from build123d import *

# Parameters (mm, degrees)
SKETCH_2_W           = 80
SKETCH_2_H           = 34
SKETCH_2_R           = 4.05
EXTRUDE_1_DEPTH      = 8
SKETCH_3_R           = 2.55
CUT_EXTRUDE_1_DEPTH  = 88.292611371
CUT_EXTRUDE_2_DEPTH  = 88.292611371
SKETCH_5_R           = 1.55
CUT_EXTRUDE_3_DEPTH  = 88.292611371
CUT_EXTRUDE_4_DEPTH  = 4.5
CUT_EXTRUDE_5_DEPTH  = 4.5
SKETCH_20_R          = 5.5
CUT_EXTRUDE_12_DEPTH = 4.5
CUT_EXTRUDE_11_DEPTH = 2
EXTRUDE_2_DEPTH      = 8


with BuildPart() as part:
    # 草图2 → 凸台-拉伸1 (new body)
    with BuildSketch(Plane.XY):
        with Locations((40, 17)):
            Rectangle(SKETCH_2_W, SKETCH_2_H)
        with Locations((7, 8)):
            Circle(SKETCH_2_R, mode=Mode.SUBTRACT)
        with Locations((40, 10)):
            Circle(SKETCH_2_R, mode=Mode.SUBTRACT)
        with Locations((73, 8)):
            Circle(SKETCH_2_R, mode=Mode.SUBTRACT)
    extrude_1 = extrude(amount=EXTRUDE_1_DEPTH)

    # 草图3 → 切除-拉伸1 (cut, through all)
    with BuildSketch(Plane.XY.offset(8)):
        with Locations((23, 8)):
            Circle(SKETCH_3_R)
        with Locations((57, 8)):
            Circle(SKETCH_3_R)
    cut_extrude_1 = extrude(amount=-CUT_EXTRUDE_1_DEPTH, mode=Mode.SUBTRACT)

    # 草图4 → 切除-拉伸2 (cut, through all)
    with BuildSketch(Plane(origin=(80, 0, 0), x_dir=(0, 0, -1), z_dir=(1, 0, 0))):
        Polygon((-1.5, 32.2), (-2.5, 32.2), (-2.5, 34), (0, 34), (0, 28.8), (-1.5, 28.8), align=None)
    cut_extrude_2 = extrude(amount=-CUT_EXTRUDE_2_DEPTH, mode=Mode.SUBTRACT)

    # 草图5 → 切除-拉伸3 (cut, through all)
    with BuildSketch(Plane.XY.offset(8)):
        with Locations((48, 10)):
            Circle(SKETCH_5_R)
        with Locations((32, 10)):
            Circle(SKETCH_5_R)
    cut_extrude_3 = extrude(amount=-CUT_EXTRUDE_3_DEPTH, mode=Mode.SUBTRACT)

    # 草图7 → 切除-拉伸4 (cut)
    with BuildSketch(Plane(origin=(0, 0, 0), x_dir=(-1, 0, 0), z_dir=(0, 0, -1))):
        with BuildLine():
            Line((-27.05, 10), (-27.05, 2.5))
            ThreePointArc((-27.05, 2.5), (-27.782233047, 0.732233047), (-29.55, 0))
            Line((-29.55, 0), (-16.45, 0))
            ThreePointArc((-16.45, 0), (-18.217766953, 0.732233047), (-18.95, 2.5))
            Line((-18.95, 2.5), (-18.95, 10))
            ThreePointArc((-18.95, 10), (-23, 14.05), (-27.05, 10))
        make_face()
        with BuildLine():
            Line((-61.05, 2.5), (-61.05, 10))
            ThreePointArc((-61.05, 10), (-57, 14.05), (-52.95, 10))
            Line((-52.95, 10), (-52.95, 2.5))
            ThreePointArc((-52.95, 2.5), (-52.217766953, 0.732233047), (-50.45, 0))
            Line((-50.45, 0), (-63.55, 0))
            ThreePointArc((-63.55, 0), (-61.782233047, 0.732233047), (-61.05, 2.5))
        make_face()
    cut_extrude_4 = extrude(amount=-CUT_EXTRUDE_4_DEPTH, mode=Mode.SUBTRACT)

    # 草图8 → 切除-拉伸5 (cut)
    with BuildSketch(Plane(origin=(0, 0, 0), x_dir=(-1, 0, 0), z_dir=(0, 0, -1))):
        with BuildLine():
            Line((-30.5, 12.85), (-49.5, 12.85))
            ThreePointArc((-49.5, 12.85), (-52.35, 10), (-49.5, 7.15))
            Line((-49.5, 7.15), (-30.5, 7.15))
            ThreePointArc((-30.5, 7.15), (-27.65, 10), (-30.5, 12.85))
        make_face()
    cut_extrude_5 = extrude(amount=-CUT_EXTRUDE_5_DEPTH, mode=Mode.SUBTRACT)

    # 草图20 → 切除-拉伸12 (cut)
    with BuildSketch(Plane(origin=(0, 0, 0), x_dir=(-1, 0, 0), z_dir=(0, 0, -1))):
        with Locations((-40, 10)):
            Circle(SKETCH_20_R)
    cut_extrude_12 = extrude(amount=-CUT_EXTRUDE_12_DEPTH, mode=Mode.SUBTRACT)

    # 草图19 → 切除-拉伸11 (cut)
    with BuildSketch(Plane(origin=(0, 0, 2.5), x_dir=(-1, 0, 0), z_dir=(0, 0, -1))):
        with BuildLine():
            Line((-25, 34), (-55.247938178, 34))
            Line((-55.247938178, 34), (-55.247938178, 33.2))
            ThreePointArc((-55.247938178, 33.2), (-54.747938178, 32.7), (-54.247938178, 33.2))
            Line((-54.247938178, 33.2), (-26, 33.2))
            ThreePointArc((-26, 33.2), (-25.5, 32.7), (-25, 33.2))
            Line((-25, 33.2), (-25, 34))
        make_face()
    cut_extrude_11 = extrude(amount=-CUT_EXTRUDE_11_DEPTH, mode=Mode.SUBTRACT)

    # 草图22 → 凸台-拉伸2 (add)
    with BuildSketch(Plane.XY.offset(8)):
        with BuildLine():
            Line((0.5, -4), (6.5, -4))
            ThreePointArc((6.5, -4), (4.5, -2), (6.5, 0))
            Line((6.5, 0), (0.5, 0))
            ThreePointArc((0.5, 0), (2.5, -2), (0.5, -4))
        make_face()
        with BuildLine():
            Line((79.5, 0), (73.5, 0))
            ThreePointArc((73.5, 0), (75.5, -2), (73.5, -4))
            Line((73.5, -4), (79.5, -4))
            ThreePointArc((79.5, -4), (77.5, -2), (79.5, 0))
        make_face()
    extrude(amount=-EXTRUDE_2_DEPTH)

    # 镜向2: 凸台-拉伸1, 切除-拉伸1, 切除-拉伸2, 切除-拉伸3, 切除-拉伸4, 切除-拉伸5, 切除-拉伸12, 切除-拉伸11 across plane
    add(extrude_1.mirror(Plane(origin=(0, -2, 0), x_dir=(0, 0, 1), z_dir=(0, -1, 0))))
    add(cut_extrude_1.mirror(Plane(origin=(0, -2, 0), x_dir=(0, 0, 1), z_dir=(0, -1, 0))), mode=Mode.SUBTRACT)
    add(cut_extrude_2.mirror(Plane(origin=(0, -2, 0), x_dir=(0, 0, 1), z_dir=(0, -1, 0))), mode=Mode.SUBTRACT)
    add(cut_extrude_3.mirror(Plane(origin=(0, -2, 0), x_dir=(0, 0, 1), z_dir=(0, -1, 0))), mode=Mode.SUBTRACT)
    add(cut_extrude_4.mirror(Plane(origin=(0, -2, 0), x_dir=(0, 0, 1), z_dir=(0, -1, 0))), mode=Mode.SUBTRACT)
    add(cut_extrude_5.mirror(Plane(origin=(0, -2, 0), x_dir=(0, 0, 1), z_dir=(0, -1, 0))), mode=Mode.SUBTRACT)
    add(cut_extrude_12.mirror(Plane(origin=(0, -2, 0), x_dir=(0, 0, 1), z_dir=(0, -1, 0))), mode=Mode.SUBTRACT)
    add(cut_extrude_11.mirror(Plane(origin=(0, -2, 0), x_dir=(0, 0, 1), z_dir=(0, -1, 0))), mode=Mode.SUBTRACT)


solid = part.part
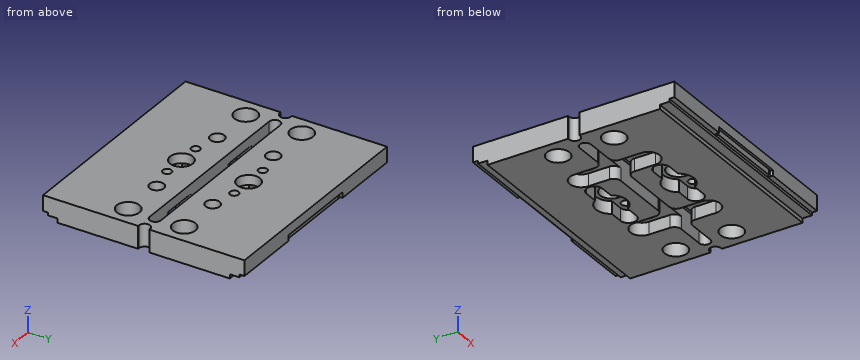
Part model, mm, in its own coordinate system. Round coordinates to 2 decimals unless told otherwise and drop trailing zeros. Order: outer loops, then holes, each group sorted by start corner. A loop starts at its lowest first (then second) coordinate and runs counter-clockwise, first axis right, second up. Notation, with made-up numbers: (44.5, 82) -> (57.5, 82) arc R25 cw to (57.5, 118) -> close; hole circle Ø5 at (34, 8.25). An arc over 180 degrees is marked (long way). Put each result on its own line as item: value.
Q1. Band-saw the part on B-B (y = -1). Give the cut face in (x, z).
From the geometry:
outline: (2.23, 0) -> (4.77, 0) -> (4.77, 8) -> (2.23, 8) -> close; (75.23, 0) -> (77.77, 0) -> (77.77, 8) -> (75.23, 8) -> close
Q2. Band-saw the part on A-A (x = 23). Give the cut face in (y, z).
From the geometry:
outline: (-38, 2.5) -> (-36.2, 2.5) -> (-36.2, 1.5) -> (-32.8, 1.5) -> (-32.8, 0) -> (-18.05, 0) -> (-18.05, 4.5) -> (-14.55, 4.5) -> (-14.55, 8) -> (-38, 8) -> close; (-9.45, 4.5) -> (-4, 4.5) -> (-4, 8) -> (-9.45, 8) -> close; (0, 4.5) -> (5.45, 4.5) -> (5.45, 8) -> (0, 8) -> close; (10.55, 4.5) -> (14.05, 4.5) -> (14.05, 0) -> (28.8, 0) -> (28.8, 1.5) -> (32.2, 1.5) -> (32.2, 2.5) -> (34, 2.5) -> (34, 8) -> (10.55, 8) -> close
Q3. Wall check: line 1 (Y direction, x = 7, z = 6.5); line 2 (Y direction, x = 32, z = 7.3); line 3 (X direction, y = -9.5, z = 1.25). Give the ranges that are in metal, low to high. Write a range as [from, to].
From the geometry:
line 1: y = [-38, -16.05], [-7.95, -4], [0, 3.95], [12.05, 34]
line 2: y = [-38, -15.55], [-12.45, -4], [0, 8.45], [11.55, 34]
line 3: x = [0, 3.81], [10.19, 18.95], [27.05, 36.84], [43.16, 52.95], [61.05, 69.81], [76.19, 80]
Q4. Pin check, flat tips, straight feed: pin 1 Ø0.5 at (x, y) = (30.5, 33) entering from -Z; pin 2 Ø5 at (x, y) = (70, -20) entering from -Z; pin 3 Ø10.5 at (x, y) = (40, -14) entering from -Z; pin 4 Ø0.8 at (x, z) = (58.5, 0.5) entering from +Y. Stop position of each tip, or through.
From the geometry:
pin 1: stops at z = 2.5
pin 2: stops at z = 0
pin 3: stops at z = 4.5
pin 4: stops at y = 28.8
Q5. Band-saw the part on C-C (x = 48). State how many separate pieces and enclosed holes the cut face has, and give its area (3 significant figures).
From the geometry:
separate pieces: 4
enclosed holes: 0
area: 449 mm2
